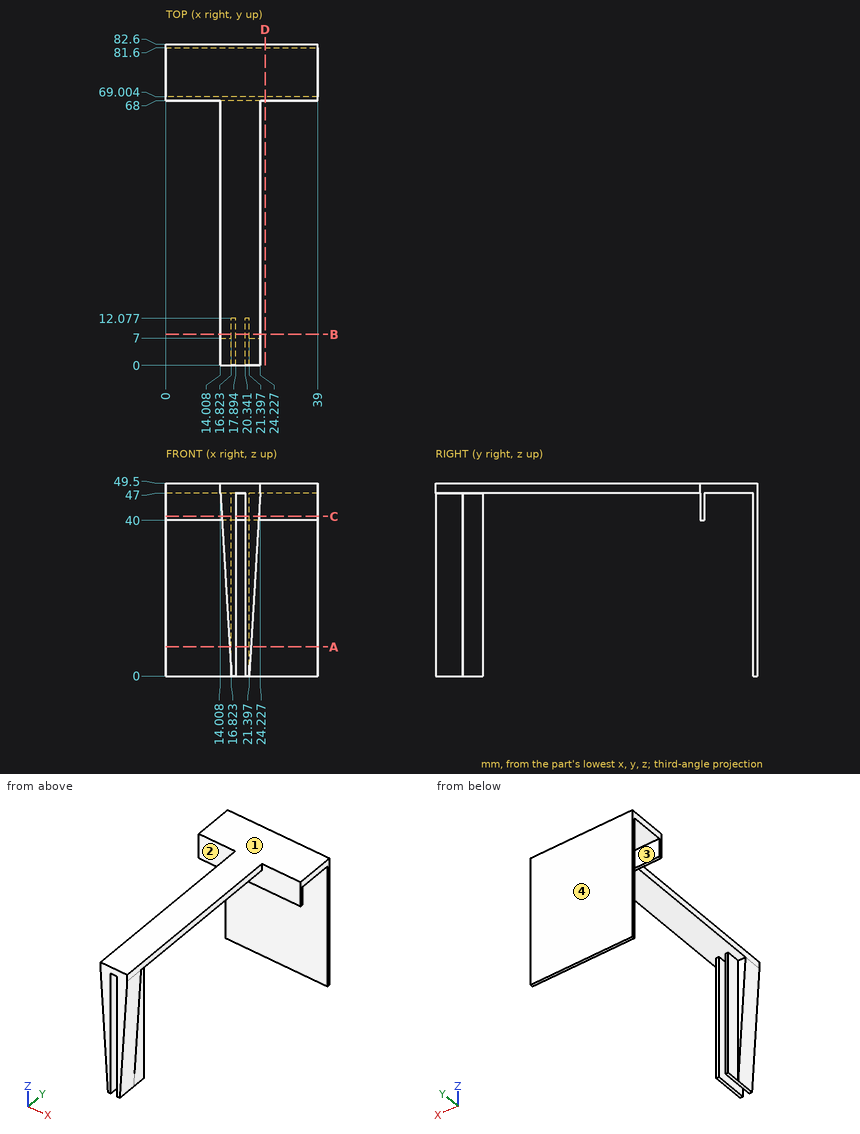
The figure shows three views and two pictorial views of one solid part (mm, origin at its lowest corner). Answer the questions. Coordinates: 2 decimals unless noted, no trailing zeros. Loops run counter-clockwise (first coordinate to the right, second up) from the corner with the lowest first, then second, coordinate; pieces in that order, holes last.
1) Determine the mould class of the marked faces 1, 2, 3 and 4 for opening direction Y: pulls with the +Y half, pulls with the -Y half, needs draft (parallel to the pull), parting line crosses it, or undercut.
2) Find section D-D on x = 25.5. Write down the section's boundary in (y, z).
3) Find section A-A on z = 7.5. Write down the section's boundary in (x, y) (1 decimal).
4) Find the intervals of material crossed by L1, parallel to Y at x = 23, z = 30; L2, parallel to Y at x = 17, z = 25.5; L3, parallel to Z at x = 29.5, y = 71.5, in increasing order.
5) Find section C-C on z = 41. Write down the section's boundary in (x, y) (1 decimal).
6) Find section B-B on y = 8. Write down the section's boundary in (x, z) (1 decimal).
7) Flat-ended cylindrical pins translate along their axes: pin 1 Ø3 at (y, z) = (9, 23) entering from -X; pin 2 Ø8 at (x, y) = (28, 30) entering from -Z; pin 3 Ø9.5 at (y, z) = (6.5, 29) entering from +X. Find the tip coordinate at first contact, or state that the pin passes through.
Values:
1. face 1: needs draft
1. face 2: undercut
1. face 3: undercut
1. face 4: pulls with the +Y half
2. outline: (68, 40) - (69, 40) - (69, 47) - (81.6, 47) - (81.6, 0) - (82.6, 0) - (82.6, 49.5) - (68, 49.5) - close
3. outline: (0, 81.6) - (39, 81.6) - (39, 82.6) - (0, 82.6) - close; (16.4, 0) - (17.9, 0) - (17.9, 12.1) - (16.8, 12.1) - (16.8, 7) - (16.4, 7) - close; (20.3, 0) - (21.8, 0) - (21.8, 7) - (21.4, 7) - (21.4, 12.1) - (20.3, 12.1) - close
4. L1: y = 0 to 7, 81.6 to 82.6
4. L2: y = 0 to 12.08, 81.6 to 82.6
4. L3: z = 47 to 49.5
5. outline: (0, 68) - (39, 68) - (39, 69) - (0, 69) - close; (0, 81.6) - (39, 81.6) - (39, 82.6) - (0, 82.6) - close; (14.4, 0) - (17.9, 0) - (17.9, 12.1) - (16.8, 12.1) - (16.8, 7) - (14.4, 7) - close; (20.3, 0) - (23.9, 0) - (23.9, 7) - (21.4, 7) - (21.4, 12.1) - (20.3, 12.1) - close
6. outline: (14, 47) - (16.8, 47) - (16.8, 0) - (17.9, 0) - (17.9, 47) - (20.3, 47) - (20.3, 0) - (21.4, 0) - (21.4, 47) - (24.2, 47) - (24.2, 49.5) - (14, 49.5) - close
7. pin 1: stops at x = 16.82
7. pin 2: stops at z = 47
7. pin 3: stops at x = 23.43
